from build123d import *

# Parameters (mm, degrees)
F0_R     = 13.562221
F1_DEPTH = 76.2
F3_D     = 6.35
F4_R     = 5.08
F5_R     = 5.08


with BuildPart() as f1:
    # F0 (on Front) → F1 (new body)
    with BuildSketch(Plane.XZ):
        with Locations((-17.780002, 21.714916)):
            Circle(F0_R)
    extrude(amount=F1_DEPTH)

    # F3 (through all)
    with Locations(Plane.XZ.offset(76.2)):
        with Locations((-17.780002, 21.714916)):
            Hole(F3_D / 2)

    # F4
    f4_edges = [f1.edges().sort_by_distance(p)[0] for p in [
        (-31.342224, -76.2, 21.714916),
    ]]
    fillet(f4_edges, radius=F4_R)

    # F5
    f5_edges = [f1.edges().sort_by_distance(p)[0] for p in [
        (-31.342224, 0, 21.714916),
    ]]
    fillet(f5_edges, radius=F5_R)


solid = f1.part
The listing builds one solid part. Answer for the finished solid, in the listing's coordinates (mm). Round coordinates to 2 decimals unless told otherwise and drop trailing zeros. Write each loop counter-clockwise with the first axis right and the second up, starting at its lowest first coordinate (ties: lowest second). Pieces come first, ordered by that corner, then holes. Notation, with made-up numbers: (74.5, 50) - (109.5, 50) arc R8 ccw to (109.5, 55) - close; hole circle Ø7 at (3, 73.25). An arc over 180 degrees is marked (long way). Use a Markdown table: item, result. Add a question column.
1. Consider line 1 (X direction, y = -25.5, z = 22.5); line 2 (Z direction, x = -17.25, y = -23); line 3 (X direction, y = -51.5, z = 24). Determine where each line is inside the solid, lowest interval first.
2. Flat-ended cylindrical pins translate along their axes: P1, Ø8, axis at x = -9, y = -10, coming from the +Z side; P2, Ø6, axis at y = -54, z = 16.5, coming from the +X side; P3, Ø2, axis at x = -27, y = -53.5, coming from the -Z side. Find the tip coordinate at first contact, or state that the pin passes through.
3. The part is cut by section A-A (y = -32.5). Write down the section's boundary in (x, z) (3 decimals).
4. For a pull along X with two mould halves and no side action, classify faces 1 (the face through (-17.367, -37.567, 24.863)), 2 (the face through (-10.49, -37.64, 33.15)), 3 (the face through (-14, 0, 22)) as +X half, -X half, draft (parallel to the pull), parting line (faces both ways), or undercut.
Reported:
| question | item | result |
|---|---|---|
| 1 | line 1 | -31.32 to -20.86, -14.7 to -4.24 |
| 1 | line 2 | 8.16 to 18.58, 24.85 to 35.27 |
| 1 | line 3 | -31.15 to -19.98, -15.58 to -4.41 |
| 2 | P1 | z = 34.41 |
| 2 | P2 | x = -4.4 |
| 2 | P3 | z = 10.93 |
| 3 | outline | circle Ø27.124 at (-17.78, 21.715); hole circle Ø6.35 at (-17.78, 21.715) |
| 4 | face 1 | undercut |
| 4 | face 2 | parting line |
| 4 | face 3 | draft |
